Source: three-view drawing plus pictorial views. Frame: mm from the lowest corner of the part. Give positions to 0.01 mm unless a question says otherwise; leave off trailing zeros. Loops run counter-clockwise (first coordinate to the right, second up) from the corner with the lowest first, then second, coordinate; pieces in that order, holes last. Notation, with made-up numbers: (-38, 23.5) -> (13, 23.5) arc R16 cw to (13, 34.5) -> close; hole circle Ø3 at (50.5, 88). An arc over 180 degrees is marked (long way). Answer in a Markdown table with one row per item. Add a question column.
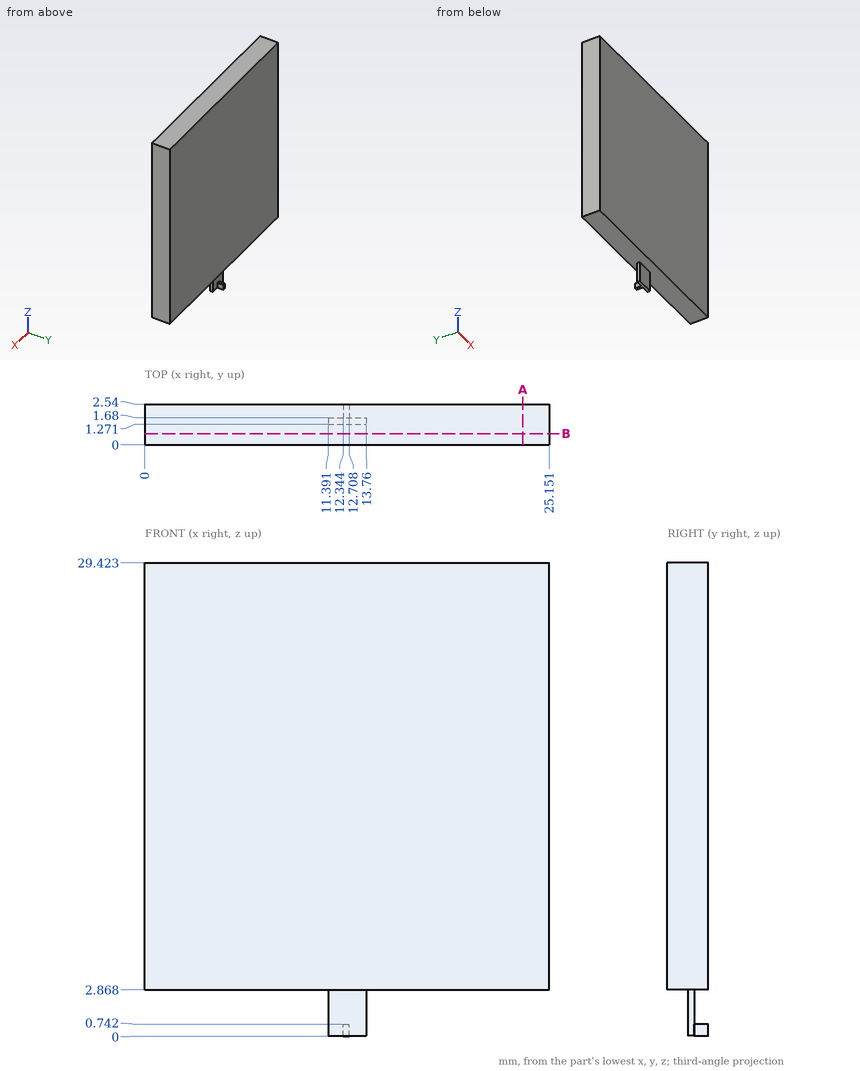
(1) Pin query (flat end, axial travel): pin 1 Ø1.2 at (x, z) = (13, 1.5) entering from -Y; pin 2 Ø0.8 at (y, z) = (2, 0.5) entering from -X; pin 3 Ø0.8 at (y, z) = (2, 0.5) entering from +X. Return the tip coordinate at first contact, or that it passes through.
(2) Material intervals for line 1 along Z through (x, y) = (18.75, 1.2), sorted ascending. Write a range as from..to.
(3) Cut plane B-B on y = 0.7. Return the cut outline in (x, z).
(4) Cut plane A-A on x = 23.5. Return the cut outline in (y, z).
Answer list:
| question | item | result |
|---|---|---|
| 1 | pin 1 | stops at y = 1.27 |
| 1 | pin 2 | stops at x = 11.39 |
| 1 | pin 3 | stops at x = 13.76 |
| 2 | line 1 | z = 2.87..29.42 |
| 3 | outline | (0, 2.87) -> (25.15, 2.87) -> (25.15, 29.42) -> (0, 29.42) -> close |
| 4 | outline | (0, 2.87) -> (2.54, 2.87) -> (2.54, 29.42) -> (0, 29.42) -> close |
